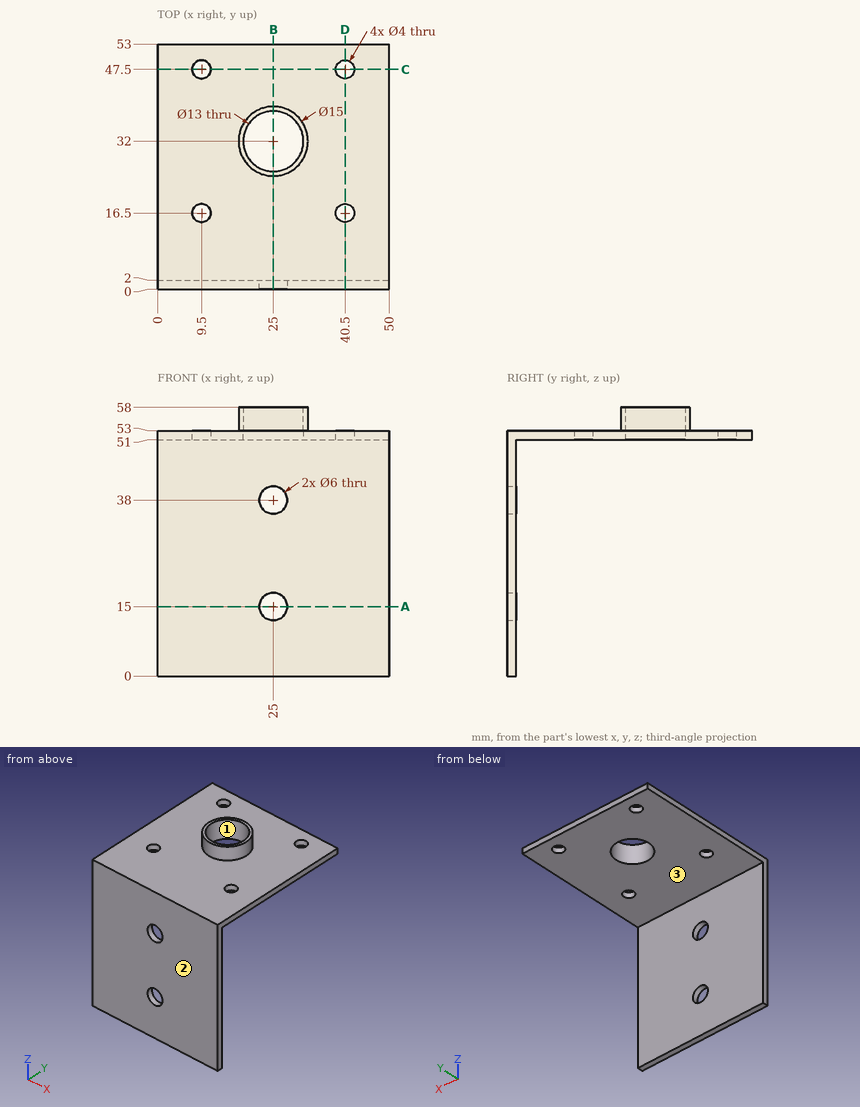
Study the drawing (mm; zero at the part's minimum x, y, z) and answer. Give positions to 0.01 mm unless a question says otherwise; leave off trailing zeros. Loops run counter-clockwise (first coordinate to the right, second up) from the corner with the lowest first, then second, coordinate; pieces in that order, holes last. Notation, with made-up numbers: (27.5, 71.25) - (70.5, 71.25) arc R15 ccw to (70.5, 80.25) - close; hole circle Ø9 at (-4.75, 32.5). An arc over 180 degrees is marked (long way). Answer as CSV lines item,"result". Start each with the question number.
1) Straight lines are drawn through the part: L1, parallel to Y at x = 9.5, z = 52.5; L2, parallel to X at y = 32, z = 52.75; L3, parallel to X at y = 1.2, z = 38. For each, find the intervals that lie inside material, in ascending order. Write a range as from..to.
2) Each of these flat-tipped pins is pushed along its axis until it touches: pin 1 Ø1 at (x, y) = (35, 41) entering from -Z; pin 2 Ø7 at (x, z) = (25, 38) entering from +Y; pin 3 Ø7 at (x, z) = (25, 15) entering from -Y; pin 4 Ø4.5 at (x, y) = (40.5, 16.5) entering from +Z. Where does it stop, or does it pass through?
3) Find section A-A (z = 15). Write down the section's boundary in (x, y).
4) Find section C-C (y = 47.5). Write down the section's boundary in (x, z).
5) Find section D-D (x = 40.5). Write down the section's boundary in (y, z).
6) Find section B-B (x = 25). Write down the section's boundary in (y, z), then the cut area to 3 significant figures.
7) Determine the mould class of the marked faces 1, 2 and 3 for opening direction Y: released by +Y, released by -Y, zero draft, split by the parting line, or undercut.
Findings below:
1,L1,"0..14.5, 18.5..45.5, 49.5..53"
1,L2,"0..18.5, 31.5..50"
1,L3,"0..22, 28..50"
2,pin 1,"z = 51"
2,pin 2,"y = 2"
2,pin 3,"y = 0"
2,pin 4,"z = 53"
3,outline,"(0, 0) - (22, 0) - (22, 2) - (0, 2) - close; (28, 0) - (50, 0) - (50, 2) - (28, 2) - close"
4,outline,"(0, 51) - (7.5, 51) - (7.5, 53) - (0, 53) - close; (11.5, 51) - (38.5, 51) - (38.5, 53) - (11.5, 53) - close; (42.5, 51) - (50, 51) - (50, 53) - (42.5, 53) - close"
5,outline,"(0, 0) - (2, 0) - (2, 51) - (14.5, 51) - (14.5, 53) - (0, 53) - close; (18.5, 51) - (45.5, 51) - (45.5, 53) - (18.5, 53) - close; (49.5, 51) - (53, 51) - (53, 53) - (49.5, 53) - close"
6,outline,"(0, 0) - (2, 0) - (2, 12) - (0, 12) - close; (0, 18) - (2, 18) - (2, 35) - (0, 35) - close; (0, 41) - (2, 41) - (2, 51) - (25.5, 51) - (25.5, 58) - (24.5, 58) - (24.5, 53) - (0, 53) - close; (38.5, 51) - (53, 51) - (53, 53) - (39.5, 53) - (39.5, 58) - (38.5, 58) - close"
6,area,"168 mm^2"
7,face 1,"undercut"
7,face 2,"released by -Y"
7,face 3,"zero draft"
